Read the model definition and answer for the solid it produces. Units are mm, in the model's axes. Face numbers are marked on the shaded views. A direction names the side the tool comes from. Give positions to 0.01 mm unless a question says otherwise; leave off trailing zeros. Order: outer loops, then holes, each group sorted by start corner. A loop starts at its lowest first (then second) coordinate and runs counter-clockwise, first axis right, second up. Notation, with made-up numbers: (-10.5, -36.5) - (18.5, -36.5) arc R14 ccw to (18.5, -18.5) - close; hole circle Ø2 at (-1.75, -19.5). An arc over 180 degrees is marked (long way). Return JSON: item names as keys, results as strings.
```python
from build123d import *

# Parameters (mm, degrees)
ESQUISSE4_W             = 100
ESQUISSE4_H             = 79
BOSS_EXTRU_3_DEPTH      = 1
BOSS_EXTRU_4_DEPTH      = 4
BOSS_EXTRU_4_DEPTH_BACK = 4
ESQUISSE1_R             = 7
ESQUISSE1_R_2           = 3.5
ESQUISSE6_R             = 11.5
BOSS_EXTRU_5_DEPTH      = 17
BOSS_EXTRU_6_DEPTH      = 1
ESQUISSE8_W             = 65
ESQUISSE8_H             = 37
ENL_V_MAT_EXTRU_1_DEPTH = 1
ESQUISSE9_R             = 1
BOSS_EXTRU_7_DEPTH      = 18
ESQUISSE10_R            = 11.5
BOSS_EXTRU_8_DEPTH      = 50
CONG_2_R                = 5
ENL_V_START             = -45
ENL_V_MAT_EXTRU_3_DEPTH = 45
ESQUISSE12_R            = 11.5
BOSS_EXTRU_9_DEPTH      = 20


with BuildPart() as part:
    # Esquisse4 → Boss.-Extru.3 (new body)
    with BuildSketch(Plane(origin=(0, 0, 0), x_dir=(1, 0, 0), z_dir=(0, 1, 0))):
        Rectangle(ESQUISSE4_W, ESQUISSE4_H)
    extrude(amount=-BOSS_EXTRU_3_DEPTH)

    # Esquisse1 → Boss.-Extru.4 (add, two sides: drawn at the far end of the back side and taken through both)
    # profile 1 of 4: a face of its own
    with BuildSketch(Plane(origin=(0, 0, 0), x_dir=(1, 0, 0), z_dir=(0, 1, 0)).offset(-BOSS_EXTRU_4_DEPTH_BACK)):
        with Locations(Location((43, 32.5, 0), (0, 0, 90))):
            Circle(ESQUISSE1_R)
        with Locations(Location((43, 32.5, 0), (0, 0, 90))):
            Circle(ESQUISSE1_R_2, mode=Mode.SUBTRACT)
    # profile 2 of 4: a face of its own
    with BuildSketch(Plane(origin=(0, 0, 0), x_dir=(1, 0, 0), z_dir=(0, 1, 0)).offset(-BOSS_EXTRU_4_DEPTH_BACK)):
        with Locations(Location((-43, 32.5, 0), (0, 0, 90))):
            Circle(ESQUISSE1_R)
        with Locations(Location((-43, 32.5, 0), (0, 0, 90))):
            Circle(ESQUISSE1_R_2, mode=Mode.SUBTRACT)
    # profile 3 of 4: a face of its own
    with BuildSketch(Plane(origin=(0, 0, 0), x_dir=(1, 0, 0), z_dir=(0, 1, 0)).offset(-BOSS_EXTRU_4_DEPTH_BACK)):
        with Locations(Location((-43, -32.5, 0), (0, 0, 270))):
            Circle(ESQUISSE1_R)
        with Locations(Location((-43, -32.5, 0), (0, 0, 90))):
            Circle(ESQUISSE1_R_2, mode=Mode.SUBTRACT)
    # profile 4 of 4: a face of its own
    with BuildSketch(Plane(origin=(0, 0, 0), x_dir=(1, 0, 0), z_dir=(0, 1, 0)).offset(-BOSS_EXTRU_4_DEPTH_BACK)):
        with Locations(Location((43, -32.5, 0), (0, 0, 270))):
            Circle(ESQUISSE1_R)
        with Locations(Location((43, -32.5, 0), (0, 0, 90))):
            Circle(ESQUISSE1_R_2, mode=Mode.SUBTRACT)
    extrude(amount=BOSS_EXTRU_4_DEPTH + BOSS_EXTRU_4_DEPTH_BACK)

    # Esquisse6 → Boss.-Extru.5 (add)
    with BuildSketch(Plane(origin=(0, 0, 0), x_dir=(1, 0, 0), z_dir=(0, 1, 0))):
        with Locations(Location((-38.5, -9.5, 0), (0, 0, 180))):
            Circle(ESQUISSE6_R)
        with Locations(Location((-15, 28, 0), (0, 0, 90))):
            Circle(ESQUISSE6_R)
    extrude(amount=BOSS_EXTRU_5_DEPTH)

    # Esquisse7 → Boss.-Extru.6 (add)
    with BuildSketch(Plane(origin=(0, 17, 0), x_dir=(1, 0, 0), z_dir=(0, 1, 0))):
        Polygon((-38.143774149, -19.88751618), (-28.414215556, -15.025120102), (-28.414215556, -3.974879898), (-22.428299765, -0.98338823), (-22.428299765, 19.221027247), (-7.571700235, 19.221027247), (-7.571700235, 34.680148422), (-13.988712335, 34.680148422), (-15.667356388, 38.039082045), (-35.613243864, 38.039082045), (-35.613243864, 23.559466539), (-38.143774149, 23.559466539), (-38.143774149, 0), align=None)
    extrude(amount=BOSS_EXTRU_6_DEPTH)

    # Esquisse8 → Enl_v. mat.-Extru.1 (cut)
    with BuildSketch(Plane(origin=(0, 0, 0), x_dir=(1, 0, 0), z_dir=(0, 1, 0))):
        with Locations((5.5, -8)):
            Rectangle(ESQUISSE8_W, ESQUISSE8_H)
    extrude(amount=-ENL_V_MAT_EXTRU_1_DEPTH, mode=Mode.SUBTRACT)

    # Esquisse9 → Boss.-Extru.7 (add)
    with BuildSketch(Plane.XZ.offset(1)):
        with Locations(Location((-40, 9.5, 0), (0, 0, 270))):
            Circle(ESQUISSE9_R)
    extrude(amount=BOSS_EXTRU_7_DEPTH)

    # Esquisse10 → Boss.-Extru.8 (add)
    with BuildSketch(Plane(origin=(0, 18, 0), x_dir=(1, 0, 0), z_dir=(0, 1, 0))):
        with Locations(Location((-38.5, -9.5, 0), (0, 0, 88.224912761))):
            Circle(ESQUISSE10_R)
    extrude(amount=BOSS_EXTRU_8_DEPTH)

    # Cong_2
    cong_2_edges = [part.edges().sort_by_distance(p)[0] for p in [
        (50, -0.5, 39.5),
        (-50, -0.5, 39.5),
        (-50, -0.5, -39.5),
        (50, -0.5, -39.5),
    ]]
    fillet(cong_2_edges, radius=CONG_2_R)

    # Esquisse11 → Enl_v. mat.-Extru.3 (cut)
    with BuildSketch(Plane(origin=(0, 68, 0), x_dir=(1, 0, 0), z_dir=(0, 1, 0)).offset(ENL_V_START)):
        with BuildLine():
            Line((-30, -17.245966692), (-30, -1.754033308))
            ThreePointArc((-30, -1.754033308), (-27, -9.5), (-30, -17.245966692))
        make_face()
    extrude(amount=ENL_V_MAT_EXTRU_3_DEPTH, mode=Mode.SUBTRACT)

    # Esquisse12 → Boss.-Extru.9 (add)
    with BuildSketch(Plane(origin=(0, 68, 0), x_dir=(1, 0, 0), z_dir=(0, 1, 0))):
        with Locations(Location((-38.5, -9.5, 0), (0, 0, 88.224912761))):
            Circle(ESQUISSE12_R)
    extrude(amount=BOSS_EXTRU_9_DEPTH)


solid = part.part
```
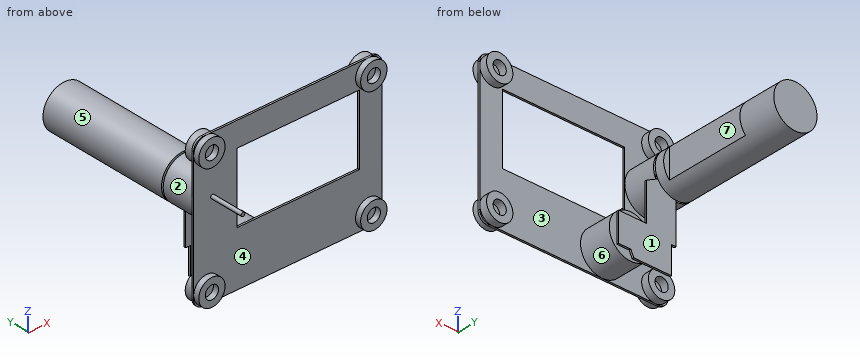
Q1. A cutting plane is placed at B-B (z = 6). Write down the section's boundary in (x, y), and give its area (3 significant figures).
Values:
{"outline": "(-50, -1) - (-27, -1) - (-27, 0) - (-27.55, 0) - (-27.55, 17) - (-28.41, 17) - (-28.41, 18) - (-27.55, 18) - (-27.55, 23) - (-30, 23) - (-30, 68) - (-27.55, 68) - (-27.55, 88) - (-49.45, 88) - (-49.45, 18) - (-38.14, 18) - (-38.14, 17) - (-49.45, 17) - (-49.45, 0) - (-50, 0) - close; (38, -1) - (50, -1) - (50, 0) - (38, 0) - close", "area": "1,840 mm²"}
Q2. A cutting plane is placed at A-A (x = 7). Write down the section's boundary in (y, z), and give its area (3 significant figures).
Values:
{"outline": "(-1, -39.5) - (0, -39.5) - (0, -10.5) - (-1, -10.5) - close; (-1, 26.5) - (0, 26.5) - (0, 39.5) - (-1, 39.5) - close", "area": "42.0 mm²"}
Q3. A cutting plane is placed at D-D (x = -33.5). Write down the section's boundary in (y, z), and give its area (3 significant figures).
Values:
{"outline": "(-1, -39.5) - (0, -39.5) - (0, -0.86) - (17, -0.86) - (17, -38.04) - (18, -38.04) - (18, -0.86) - (88, -0.86) - (88, 19.86) - (18, 19.86) - (18, 17.57) - (17, 17.57) - (17, 19.86) - (0, 19.86) - (0, 39.5) - (-1, 39.5) - close", "area": "1,940 mm²"}
Q4. Determine the mould class of the marked faces 1, 2, 3 and 4 for opening direction X: released by +X, released by -X, zero draft, split by the parting line, or undercut.
Values:
{"face 1": "zero draft", "face 2": "split by the parting line", "face 3": "undercut", "face 4": "undercut"}
Q5. A cutting plane is placed at C-C (y = 10). Write down the section's boundary in (x, z), and give its area (3 significant figures).
Values:
{"outline": "circle Ø23 at (-38.5, 9.5); circle Ø23 at (-15, -28)", "area": "831 mm²"}
Q6. Given pin 1 (5 mm diameter, centred on x = -36.5, y = 56, fed in from -Z); pin 2 (7.5 mm diameter, centred on x = -41.5, z = -32, fed in from -Y); pin 3 (0.8 mm diameter, centred on x = -37, y = 17.5, fed in from -Z), each flat-ended and moving along its own axis, determine where each tip first touches the part or whether it passes through.
Values:
{"pin 1": "stops at z = -2", "pin 2": "stops at y = -4", "pin 3": "stops at z = -23.56"}
Q7. For the marked faces 5, 6 and 7, determine the directions among +Z, -Z, +X, -X, +Y, -Y from which every point of the face is accessible in a straight line to the end or side of a thin tool.
Values:
{"face 5": "+Y", "face 6": "none", "face 7": "+Z, -Z, +X"}
Q8. Consider L1, parallel to X at y = -2.8, z = 32.5; L2, parallel to Z at x = 43, y = -2; L3, parallel to X at y = 1, z = -32. Determine where each line is inside the solid, lowest interval first.
Values:
{"L1": "x = -50 to -46.5, -39.5 to -36, 36 to 39.5, 46.5 to 50", "L2": "z = -39.5 to -36, -29 to -25.5, 25.5 to 29, 36 to 39.5", "L3": "x = -49.98 to -46.46, -39.54 to -36.02, -25.78 to -4.22, 36.02 to 39.54, 46.46 to 49.98"}
